Input: dimensioned drawing with shaded views. Units: mm. Origin: part minimum x, y, z. Round coordinates to 2 decimals unless told otherwise and drop trailing zeros. Put each result on its own line as item: value. Start each with the question number.
1) Line query: probe 1 along X at (y, z) = (4.5, 5.08) (1 decimal); probe 2 along X at (y, z) = (2.25, 5.08); probe 3 along Y at (x, z) = (14.5, 32.5) (1 decimal). Output: solid intervals per line, ascending.
2) Pin query (flat end, axial travel): pin 1 (1 mm diameter, centred on x = 23, y = 5, fed in from +Z); pin 2 (1.6 mm diameter, centred on y = 4.5, z = 23, fed in from +X) (1 decimal); pin 3 (3 mm diameter, centred on x = 18, z = 23, fed in from +Y) (1 decimal). Return the tip coordinate at first contact, or that it passes through.
3) Draft query along X for the marked faces 1 and 2. Return one class per face: +X half, -X half, draft (parallel to the pull), parting line (faces both ways), or undercut.
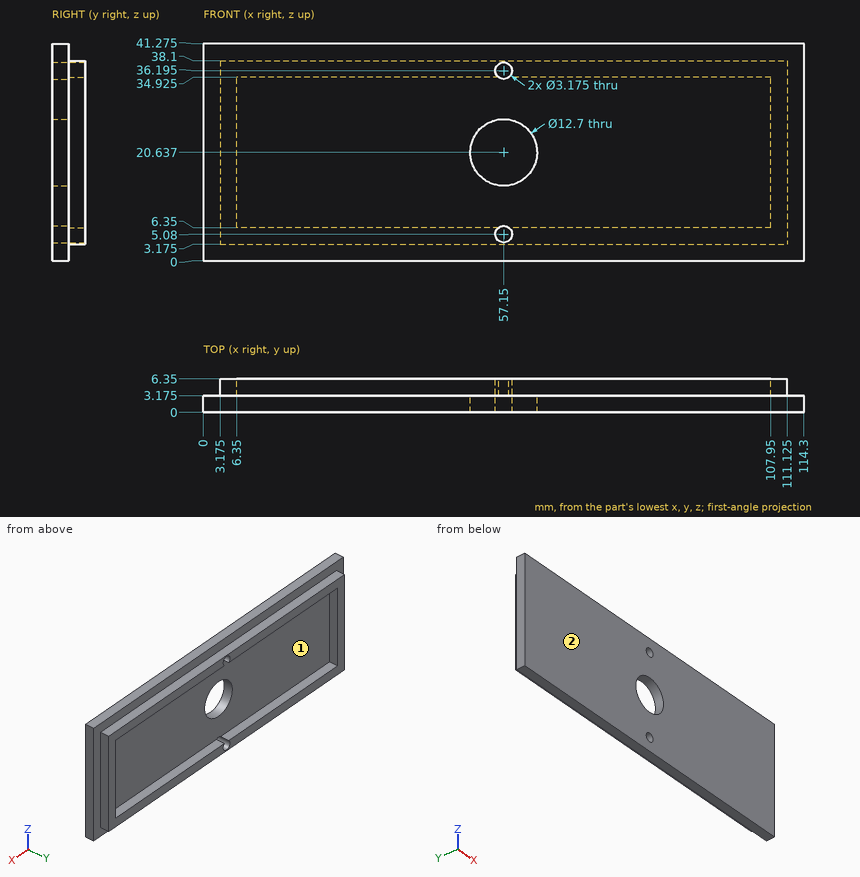
Geometry results:
1. probe 1: x = 3.2 to 55.6, 58.7 to 111.1
1. probe 2: x = 0 to 55.56, 58.74 to 114.3
1. probe 3: y = 0 to 3.2
2. pin 1: stops at z = 38.1
2. pin 2: stops at x = 111.1
2. pin 3: stops at y = 3.2
3. face 1: undercut
3. face 2: draft
